Source: CAD feature listing. Evaluate the final solid. Frame: model axes, mm. Face numbers are marked on the shaded views. A direction names the side the tool comes from. Give positions to 0.01 mm unless a question says otherwise; leave off trailing zeros. Order: outer loops, then holes, each group sorted by start corner. A loop starts at its lowest first (then second) coordinate and runs counter-clockwise, first axis right, second up. Notation, with made-up numbers: M 63,87 L 95,87 A24 cw 95,125 Z; hole C -11.75,-35.5 d10. An arc over 180 degrees is marked long. Answer as a JSON object with one key per item and string values. Group by question number.
1. Section query B-B (z = 4.25). Output: boundary loops of the cut face in (x, y) (3 decimals), plus the area to 3 significant figures.
2. Section query D-D (y = 0.25). Output: boundary loops of the cut face in (x, z), plus the area to 3 significant figures.
3. Section query A-A (x = 5). Output: boundary loops of the cut face in (y, z), plus the area to 3 significant figures.
4. Material intervals for L1, parallel to Y at x = 1.5, z = 3; L2, parallel to X at y = -1.5, z = 3.5; L3, parallel to X at y = -2, z = 5.5, sorted ascending. Write a range as [from, to].
5. Pin query (flat end, axial travel): P1, Ø1, axis at x = 45.5, z = 4, coming from the -Y side; P2, Ø1.1, axis at y = 8, z = 3.5, coming from the -X side; P3, Ø3, axis at y = 0.5, z = 4, coming from the +X side; P4, Ø1.4, axis at x = 3.02, y = -1.92, coming from the +Z side. Return the tip coordinate at first contact, or that it passes through.
6. Set-up query: the marked faces 4 and 5. Return all of +Z, -Z, +X, -X, +Y, -Y with unobstructed straight access to the full face (end or side cutting, diameter ignored); none if empty.
7. Pull-direction query (Y, two-part tool) for the marked faces 1, 2 and 3; classes: +Y half, -Y half, draft (parallel to the pull), parting line (faces both ways), or undercut.
8. Section query C-C (x = -6). Output: boundary loops of the cut face in (y, z).
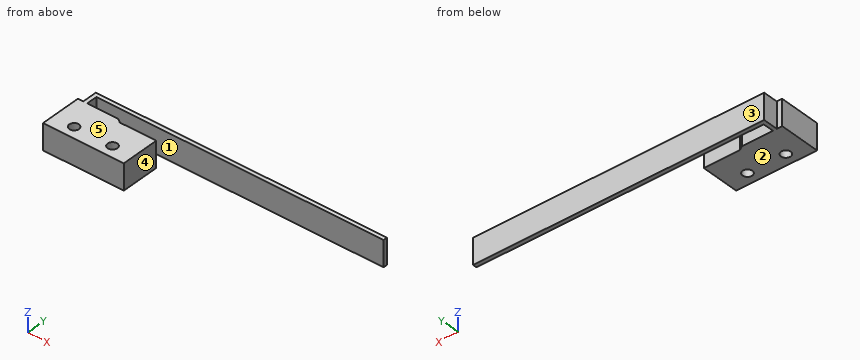
Autodesk Inventor part; units mm, degrees
ref_plane "YZ Plane" through (0, 0, 0) normal (1, 0, 0) x (0, 1, 0)
ref_plane "XZ Plane" through (0, 0, 0) normal (0, 1, 0) x (-1, 0, 0)
ref_plane "XY Plane" through (0, 0, 0) normal (0, 0, 1) x (1, 0, 0)
sketch "Sketch1" plane through (0, 0, 0) normal (0, 0, 1) x (1, 0, 0)
  line L0 (8.268, 4.6844) -> (8.268, -4.8156)
  line L1 (8.268, -4.8156) -> (-11.732, -4.8156)
  line L2 (-11.732, -4.8156) -> (-11.732, 5.3844)
  circle A0 centre (-6.482, -1.9156) radius 1.2
  circle A1 centre (3.018, -1.9156) radius 1.2
  line L3 (-9.425, 5.3844) -> (-9.425, 8.0844)
  line L4 (-9.425, 8.0844) -> (61.6567, 8.0844)
  line L5 (61.6567, 8.0844) -> (61.6567, 9.0844)
  line L6 (61.6567, 9.0844) -> (-10.3988, 9.0844)
  line L7 (-10.3988, 9.0844) -> (-10.3988, 5.3844)
  line L8 (-1.732, 5.3844) -> (-0.7437, 4.6844)
  line L9 (-0.7437, 4.6844) -> (8.268, 4.6844)
  line L10 (-11.732, 5.3844) -> (-10.3988, 5.3844)
  line L11 (-9.425, 5.3844) -> (-1.732, 5.3844)
  point P0 (0, 0)
  dimension "d0" = 20
  dimension "d2" = 2.4
  dimension "d3" = 2.4
  dimension "d4" = 9.5
  dimension "d5" = 5.25
  dimension "d6" = 2.9
  dimension "d7" = 2.9
  dimension "d8" = 10
  dimension "d9" = 11
  dimension "d10" = 9.5
extrude "Extrusion1" add sketch "Sketch1" along normal blind 6.4
equation "\"d3\" = d2"
equation "\"d7\" = d6"
properties part number "switch"
Answer sheet:
{
 "1": {"outline": "M -11.732,-4.816 L 8.268,-4.816 L 8.268,4.684 L -0.744,4.684 L -1.732,5.384 L -9.425,5.384 L -9.425,8.084 L 61.657,8.084 L 61.657,9.084 L -10.399,9.084 L -10.399,5.384 L -11.732,5.384 Z; hole C -6.482,-1.916 d2.4; hole C 3.018,-1.916 d2.4", "area": "263 mm^2"},
 "2": {"outline": "M -11.73,0 L 8.27,0 L 8.27,6.4 L -11.73,6.4 Z", "area": "128 mm^2"},
 "3": {"outline": "M -4.82,0 L 4.68,0 L 4.68,6.4 L -4.82,6.4 Z; M 8.08,0 L 9.08,0 L 9.08,6.4 L 8.08,6.4 Z", "area": "67.2 mm^2"},
 "4": {"L1": "[-4.82, 4.68], [8.08, 9.08]", "L2": "[-11.73, -7.61], [-5.36, 1.89], [4.14, 8.27]", "L3": "[-11.73, -7.68], [-5.28, 1.82], [4.22, 8.27]"},
 "5": {"P1": "y = 8.08", "P2": "x = -10.4", "P3": "x = 8.27", "P4": "through"},
 "6": {"face 4": "+Z, -Z, +X, -Y", "face 5": "+Z, +X, -X, +Y, -Y"},
 "7": {"face 1": "undercut", "face 2": "draft", "face 3": "+Y half"},
 "8": {"outline": "M -4.82,0 L -3.01,0 L -3.01,6.4 L -4.82,6.4 Z; M -0.82,0 L 5.38,0 L 5.38,6.4 L -0.82,6.4 Z; M 8.08,0 L 9.08,0 L 9.08,6.4 L 8.08,6.4 Z"}
}
